The listing builds one solid part. Answer for the finished solid, in the listing's coordinates (mm). Face numbers are marked on the shaded views. Coordinates: 2 decimals unless noted, no trailing zeros. Order: outer loops, then holes, each group sorted by start corner. A loop starts at its lowest first (then second) coordinate and runs counter-clockwise, first axis right, second up. Notation, with made-up numbers: (73.25, 31) -> (93.25, 31) arc R16 ccw to (93.25, 38) -> close; hole circle Ø8 at (75.5, 60.25). An arc over 180 degrees is marked (long way). Write item = value, one per line. Start each with the question number.
Autodesk Inventor part; units mm, degrees
ref_plane "Work Plane1" through (5.25, 0, -7.62) normal (1, 0, 0) x (0, 1, 0)
ref_plane "YZ Plane" through (0, 0, 0) normal (1, 0, 0) x (0, 1, 0)
ref_plane "XZ Plane" through (0, 0, 0) normal (0, 1, 0) x (-1, 0, 0)
sketch "Sketch1" plane through (0, 0, 0) normal (0, 0, 1) x (1, 0, 0)
  circle A0 centre (0, 0) radius 28.3972
  dimension "d0" = 56.7944
extrude "Extrusion1" add sketch "Sketch1" along normal blind 5.9944
sketch "Sketch2" plane through (0, 0, 5.9944) normal (0, 0, 1) x (1, 0, 0)
  point P0 (0, 0)
  point P1 (0, 0)
hole "Hole1" at (0, 0, 5.9944) direction (0, 0, -1) diameter 6.35 depth 5.9944
sketch "Sketch3" plane through (0, 0, 0) normal (0, 0, -1) x (-1, 0, 0)
  circle A0 centre (0, 0) radius 3.175 construction
  line L0 (0, 0) -> (0, 23.749) construction
  dimension "d10" = 23.749
hole "Hole2" at (0, 23.749, 0) direction (0, 0, 1) diameter 3.302 depth 12.2936 tip angle 118
pattern_circular "Circular Pattern1" count 6 over 360 about axis through (0, 0, 2.9972) along (0, 0, 1) of "Hole2"
sketch "Sketch4" plane through (0, 0, 5.9944) normal (0, 0, 1) x (1, 0, 0)
  circle A0 centre (0, 0) radius 3.175
  circle A1 centre (0, 0) radius 11.9888
  dimension "d22" = 23.9776
extrude "Extrusion2" add sketch "Sketch4" along normal blind 1.905
sketch "Sketch5" plane through (0, 0, 0) normal (0, 0, -1) x (-1, 0, 0)
  circle A0 centre (0, 0) radius 5.25
  circle A1 centre (0, 0) radius 3.175
  dimension "d25" = 10.5
extrude "Extrusion3" add sketch "Sketch5" along normal blind 7.62
sketch "Sketch6" plane through (0, 0, -7.62) normal (0, 0, -1) x (-1, 0, 0)
  circle A0 centre (0, 0) radius 5.25
  point P0 (-5.25, 0)
ref_plane "Work Plane1" through (5.25, 0, -7.62) normal (1, 0, 0) x (0, 1, 0)
sketch "Sketch7" plane through (5.25, 0, -7.62) normal (1, 0, 0) x (0, 1, 0)
  line L0 (0, 0) -> (0, 3.81) construction
  point P0 (0, 7.62)
  dimension "d28" = 3.81
hole "Hole3" at (5.25, 0, -3.81) direction (-1, 0, 0) diameter 3.9624 depth 6.35 tip angle 118
properties part number "Mecanum Wheel Adapter Plate"
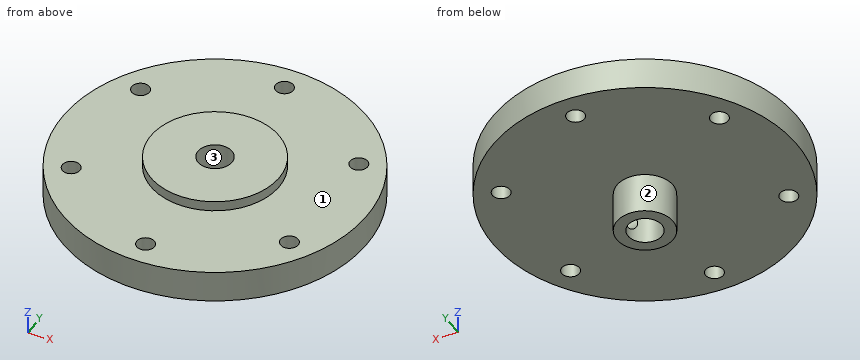
Item 1: Each of these flat-tipped pins is pushed along its axis until it touches: pin 1 (2 mm diameter, centred on x = 0, y = 23.749, fed in from +Z); pin 2 (5.5 mm diameter, centred on x = 20.57, y = 11.87, fed in from +Z); pin 3 (17 mm diameter, centred on x = -4, y = 12, fed in from +Z); pin 4 (3.5 mm diameter, centred on y = 0, z = -3.81, fed in from +X). Where does it stop, or does it pass through?
Item 2: For a pull along Y with two mould halves and no side action, classify the marked faces 1, 2 and 3 as pulls with the +Y half, pulls with the -Y half, needs draft (parallel to the pull), parting line crosses it, or undercut.
Item 3: Consider probe 1 along X at (y, z) = (0, -0.75) (3 decimals); probe 2 along Y at (x, z) = (21, 3.75); probe 3 along Z at (x, y) = (-22, -9). Determine where each line is inside the solid, lowest interval first.
Item 4: Section C-C, the plane x = -20 is taken. Give the vertices of the cut face in (y, z) (3 decimals).
Item 5: Section D-D, the plane z = 4 is taken. Give the number of separate pieces and of enclosed holes in the cut face, then the cut area to 3 significant figures.
Item 6: Section B-B, the plane y = 0 is taken. Give the vertices of the cut face in (x, z) (3 decimals), then the cut area to 3 significant figures.
Item 7: Section A-A, the plane x = 0 is taken. Give the vertices of the cut face in (y, z) (3 decimals), then the cut area to 3 significant figures.
A:
q1.pin_1 = through
q1.pin_2 = 5.99
q1.pin_3 = 7.9
q1.pin_4 = -2.65
q2.face_1 = needs draft
q2.face_2 = parting line crosses it
q2.face_3 = undercut
q3.probe_1 = -5.25 to -3.175, 3.175 to 5.25
q3.probe_2 = -19.12 to -13.47, -10.28 to 10.28, 13.47 to 19.12
q3.probe_3 = 0 to 5.99
q4.outline = (-20.159, 0) -> (-13.425, 0) -> (-13.425, 5.994) -> (-20.159, 5.994) -> close; (-10.324, 0) -> (10.324, 0) -> (10.324, 5.994) -> (-10.324, 5.994) -> close; (13.425, 0) -> (20.159, 0) -> (20.159, 5.994) -> (13.425, 5.994) -> close
q5.separate_pieces = 1
q5.enclosed_holes = 7
q5.area = 2,450 mm^2
q6.outline = (-28.397, 0) -> (-5.25, 0) -> (-5.25, -7.62) -> (-3.175, -7.62) -> (-3.175, 7.899) -> (-11.989, 7.899) -> (-11.989, 5.994) -> (-28.397, 5.994) -> close; (3.175, -7.62) -> (5.25, -7.62) -> (5.25, -5.791) -> (3.175, -5.791) -> close; (3.175, -1.829) -> (5.25, -1.829) -> (5.25, 0) -> (28.397, 0) -> (28.397, 5.994) -> (11.989, 5.994) -> (11.989, 7.899) -> (3.175, 7.899) -> close
q6.area = 359 mm^2
q7.outline = (-28.397, 0) -> (-25.4, 0) -> (-25.4, 5.994) -> (-28.397, 5.994) -> close; (-22.098, 0) -> (-5.25, 0) -> (-5.25, -7.62) -> (-3.175, -7.62) -> (-3.175, 7.899) -> (-11.989, 7.899) -> (-11.989, 5.994) -> (-22.098, 5.994) -> close; (3.175, -7.62) -> (5.25, -7.62) -> (5.25, 0) -> (22.098, 0) -> (22.098, 5.994) -> (11.989, 5.994) -> (11.989, 7.899) -> (3.175, 7.899) -> close; (25.4, 0) -> (28.397, 0) -> (28.397, 5.994) -> (25.4, 5.994) -> close
q7.area = 328 mm^2
